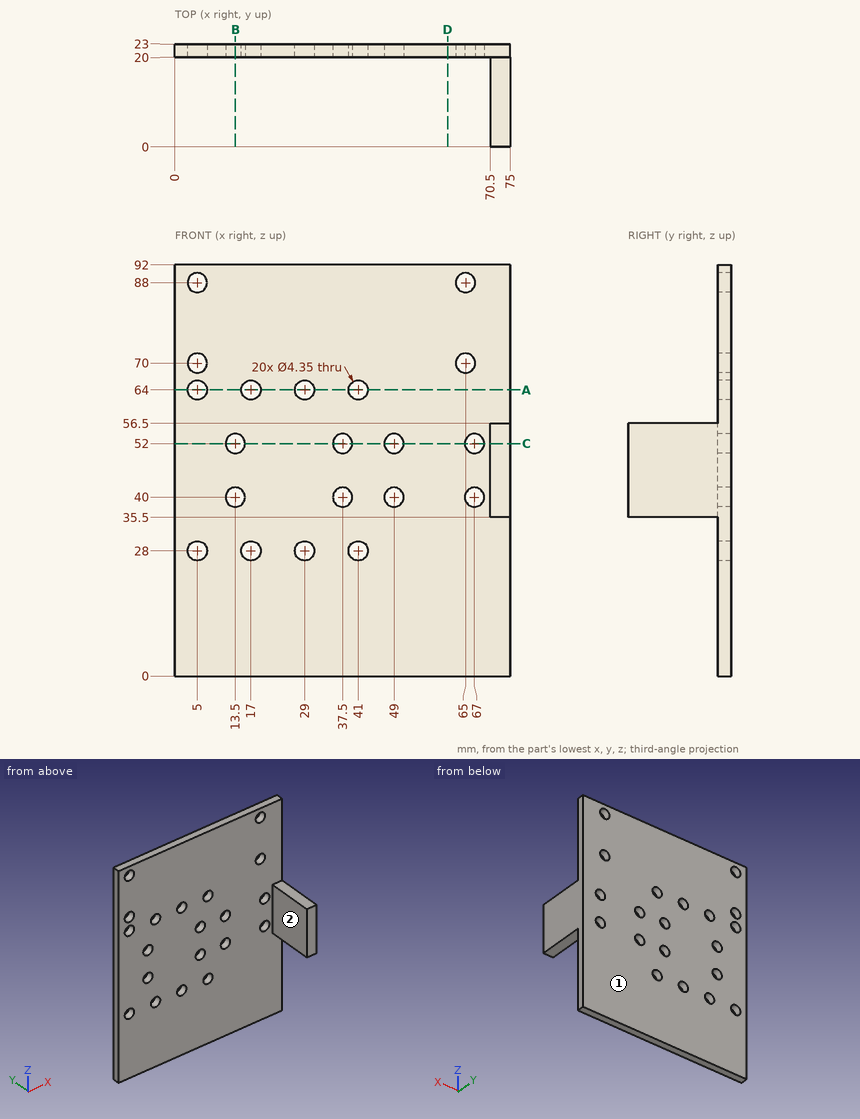
Check sheet for the drawn part. Datum: minimum x, y, z corner. Units: mm. A direction names the side the tool comes from. Give positions to 0.01 mm unless a question says otherwise; leave off trailing zeros. Loops run counter-clockwise (first coordinate to the right, second up) from the corner with the lowest first, then second, coordinate; pieces in that order, holes last.
1) Sectioned sample at B-B, the plane x = 13.5. Enter the section's corners in (y, z) (3 decimals), then the cut area to 3 significant figures.
2) Sectioned sample at A-A, the plane z = 64. Enter the section's corners in (x, y) (3 decimals), then the cut area to 3 significant figures.
3) Sectioned sample at D-D, the plane x = 61. Enter the section's corners in (y, z), then the cut area to 3 significant figures.
4) Sectioned sample at C-C, the plane z = 52. Enter the section's corners in (x, y) (3 decimals), then the cut area to 3 significant figures.
5) Depth check by flat-ended pin: pin 1 Ø7 at (x, z) = (37.5, 40) entering from +Y; pin 2 Ø1.5 at (x, z) = (62, 80.5) entering from -Y; pin 3 Ø3.5 at (x, z) = (5, 70) entering from +Y; pin 4 Ø10 at (y, z) = (12, 51) entering from -X. Enter the tip coordinate at first touch or a pass-through.
6) Set-up check for the marked faces 1 and 2: record each of +Z, -Z, +X, -X, +Y, -Y from which the full face is reachable in a straight line by a thin tool's end or side.
7) Thickness scan on line 1 along Z through (x, y) = (49, 21.4) (3 decimals); line 2 along Z through (x, y) = (5, 21.7) (3 decimals); line 3 along X through (y, z) = (21.85, 40) (3 decimals). Record the ranges inside material, lowest first.
Answers:
1. outline: (20, 0) - (23, 0) - (23, 37.825) - (20, 37.825) - close; (20, 42.175) - (23, 42.175) - (23, 49.825) - (20, 49.825) - close; (20, 54.175) - (23, 54.175) - (23, 92) - (20, 92) - close
1. area: 250 mm2
2. outline: (0, 20) - (2.825, 20) - (2.825, 23) - (0, 23) - close; (7.175, 20) - (14.825, 20) - (14.825, 23) - (7.175, 23) - close; (19.175, 20) - (26.825, 20) - (26.825, 23) - (19.175, 23) - close; (31.175, 20) - (38.825, 20) - (38.825, 23) - (31.175, 23) - close; (43.175, 20) - (75, 20) - (75, 23) - (43.175, 23) - close
2. area: 173 mm2
3. outline: (20, 0) - (23, 0) - (23, 92) - (20, 92) - close
3. area: 276 mm2
4. outline: (0, 20) - (11.325, 20) - (11.325, 23) - (0, 23) - close; (15.675, 20) - (35.325, 20) - (35.325, 23) - (15.675, 23) - close; (39.675, 20) - (46.825, 20) - (46.825, 23) - (39.675, 23) - close; (51.175, 20) - (64.825, 20) - (64.825, 23) - (51.175, 23) - close; (69.175, 20) - (70.5, 20) - (70.5, 0) - (75, 0) - (75, 23) - (69.175, 23) - close
4. area: 263 mm2
5. pin 1: stops at y = 23
5. pin 2: stops at y = 20
5. pin 3: passes through
5. pin 4: stops at x = 70.5
6. face 1: +Z, -Z, +X, -X, +Y
6. face 2: +Z, -Z, -X, -Y
7. line 1: z = 0 to 37.825, 42.175 to 49.825, 54.175 to 92
7. line 2: z = 0 to 25.825, 30.175 to 61.825, 66.175 to 67.825, 72.175 to 85.825, 90.175 to 92
7. line 3: x = 0 to 11.325, 15.675 to 35.325, 39.675 to 46.825, 51.175 to 64.825, 69.175 to 75
